Geometry check sheet. Reference: the model listing, model coordinates, mm. Face numbers are marked on the shaded views. A direction names the side the tool comes from. Give positions to 0.01 mm unless a question says otherwise; leave off trailing zeros. Order: outer loops, then holes, each group sorted by start corner. A loop starts at its lowest first (then second) coordinate and runs counter-clockwise, first axis right, second up. Notation, with made-up numbers: M 64,-0.5 L 114,-0.5 A10 cw 114,17.5 Z; hole C 80,78.5 d8. An arc over 180 degrees is marked long. Put each result on its own line as item: value. Start each with the question number.
Q1. Material ranges on L1, parallel to X at y = 10.75, z = 9.5; L2, parallel to Z at x = -13, y = 10; L3, parallel to X at y = 8.25, z = 7.75, recorded low to high.
Q2. Mould release check, pull along X, two halves, no side actions. Record for the marked faces 1, 2 and 3: +X half, -X half, draft (parallel to the pull), parting line (faces both ways), or undercut.
Q3. Go/stop test with flat-tipped pins: pin 1 (5.5 mm diameter, centred on x = 12, y = 5, fed in from +Z); pin 2 (2 mm diameter, centred on y = 8, z = 7, fed in from +X); pin 3 (4 mm diameter, centred on y = 4, z = 8, fed in from -X). Record where each tip stops, or that it passes through.
Q4. Section check A-A on z = 10.5. Record the cut outline in (x, y).
Q5. Section check D-D on y = 5. Record the cut outline in (x, z), then the cut area to 4 significant figures.
Q6. Section check B-B on x = -14. Record the cut outline in (y, z), then the cut area to 3 significant figures.
Q7. Section check C-C on y = 9.75. Record the cut outline in (x, z).
Q8. Access from +Z, -Z, +X, -X, +Y, -Y to the whole of each face (thin tool, end or side, straight path). Record for the marked faces 4, 5 and 6.
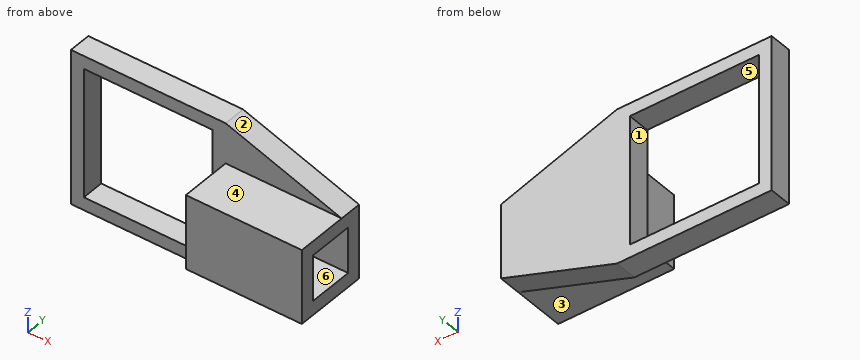
Autodesk Fusion 360 part; units mm, degrees
sketch "Sketch1" plane through (0, 0, 0) normal (0, 1, 0) x (1, 0, 0)
  line L0 (0, 0) -> (0, -11.5)
  line L1 (0, -11.5) -> (18, -11.5)
  line L2 (0, 0) -> (18, 0)
  line L3 (18, -11.5) -> (18, 0)
  dimension "d1" = 11.5
  dimension "d2" = 18
  dimension "d3" = 18
extrude "Extrude1" add sketch "Sketch1" along normal blind 11.5
sketch "Sketch2" plane through (18, 0, 0) normal (1, 0, 0) x (0, 1, 0)
  line L0 (0, 11.5) -> (0, 0)
  line L1 (0, 0) -> (11.5, 0)
  line L2 (11.5, 0) -> (11.5, 11.5)
  line L3 (11.5, 11.5) -> (0, 11.5)
  line L4 (0, 11.5) -> (0, 9.3)
  line L5 (0, 9.3) -> (2.2, 9.3)
  line L6 (2.2, 9.3) -> (9.3, 9.3)
  line L7 (9.3, 9.3) -> (9.3, 2.2)
  line L8 (9.3, 2.2) -> (2.2, 2.2)
  line L9 (2.2, 2.2) -> (2.2, 9.3)
  dimension "d9" = 2.2
  dimension "d10" = 2.2
  dimension "d11" = 7.1
  dimension "d12" = 7.1
extrude "Extrude2" cut sketch "Sketch2" against normal blind 15 contours L6 L7 L8 L9
sketch "Sketch3" plane through (0, 0, 0) normal (-1, 0, 0) x (0, -1, 0)
  line L0 (0, 0) -> (0, 11.5)
  line L1 (0, 11.5) -> (-11.5, 11.5)
  line L2 (-11.5, 11.5) -> (-11.5, 0)
  line L3 (-11.5, 0) -> (0, 0)
  line L4 (-11.5, 11.5) -> (-7.25, 11.5)
  line L5 (-7.25, 11.5) -> (-7.25, 7.25)
  line L6 (-7.25, 7.25) -> (-4.25, 7.25)
  line L7 (-4.25, 7.25) -> (-4.25, 4.25)
  line L8 (-4.25, 4.25) -> (-7.25, 4.25)
  line L9 (-7.25, 4.25) -> (-7.25, 7.25)
  dimension "d15" = 4.25
  dimension "d16" = 4.25
  dimension "d17" = 3
  dimension "d18" = 3
sketch "Sketch4" plane through (0, 0, 0) normal (-1, 0, 0) x (0, -1, 0)
  line L0 (0, 0) -> (0, 11.5)
  line L1 (0, 11.5) -> (-11.5, 11.5)
  line L2 (-11.5, 11.5) -> (-11.5, 0)
  line L3 (-11.5, 0) -> (0, 0)
  line L4 (-11.5, 11.5) -> (-11.5, 7.5)
  line L5 (-11.5, 7.5) -> (0, 7.5)
  line L6 (0, 7.5) -> (0, 4)
  line L7 (0, 4) -> (-11.5, 4)
  line L8 (-11.5, 4) -> (-11.5, 7.5)
  dimension "d21" = 4
  dimension "d22" = 3.5
sketch "Sketch5" plane through (0, 0, 0) normal (0, -1, 0) x (1, 0, 0)
  line L0 (0, 11.5) -> (0, 0)
  line L1 (0, 0) -> (18, 0)
  line L2 (18, 0) -> (18, 11.5)
  line L3 (18, 11.5) -> (0, 11.5)
  line L4 (0, 11.5) -> (0, 0)
sketch "Sketch6" plane through (0, 11.5, 0) normal (0, 1, 0) x (-1, 0, 0)
  line L0 (0, 0) -> (0, 11.5)
  line L1 (0, 11.5) -> (-18, 11.5)
  line L2 (-18, 11.5) -> (-18, 0)
  line L3 (-18, 0) -> (0, 0)
  line L4 (0, 5.75) -> (24, 5.75)
  line L5 (24, 5.75) -> (24, 17.75)
  line L6 (24, 17.75) -> (0, 17.75)
  line L7 (0, 17.75) -> (0, 5.75)
  line L8 (0, 5.75) -> (-18, 5.75) construction
  line L9 (24, 5.75) -> (24, -6.25)
  line L10 (24, -6.25) -> (0, -6.25)
  line L11 (0, 5.75) -> (24, 5.75)
  line L12 (0, -6.25) -> (0, 0)
  dimension "d26" = 24
  dimension "d27" = 12
extrude "Extrude5" add sketch "Sketch6" against normal blind 3.5 contours L0 L4 L9 L10 L11 L12 | L0 L4 L5 L6 L7 L11
sketch "Sketch7" plane through (0, 11.5, 0) normal (0, 1, 0) x (-1, 0, 0)
  line L0 (0, 11.5) -> (-18, 11.5)
  line L1 (-18, 11.5) -> (-18, 0)
  line L2 (-18, 0) -> (0, 0)
  line L3 (0, 0) -> (0, -6.25)
  line L4 (0, -6.25) -> (24, -6.25)
  line L5 (24, -6.25) -> (24, 17.75)
  line L6 (24, 17.75) -> (0, 17.75)
  line L7 (0, 17.75) -> (0, 11.5)
  line L8 (24, -6.25) -> (24, -4.25)
  line L9 (24, -4.25) -> (22, -4.25)
  line L10 (22, -4.25) -> (2, -4.25)
  line L11 (2, -4.25) -> (2, 15.75)
  line L12 (2, 15.75) -> (22, 15.75)
  line L13 (22, 15.75) -> (22, -4.25)
  dimension "d30" = 2
  dimension "d31" = 2
  dimension "d32" = 20
  dimension "d33" = 20
extrude "Extrude6" cut sketch "Sketch7" against normal blind 5 contours L10 L11 L12 L13
sketch "Sketch8" plane through (0, 0, 0) normal (1, 0, 0) x (0, 1, 0)
sketch "Sketch9" plane through (0, 11.5, 0) normal (0, 1, 0) x (-1, 0, 0)
  line L0 (2, -4.25) -> (2, 15.75)
  line L1 (2, 15.75) -> (22, 15.75)
  line L2 (22, 15.75) -> (22, -4.25)
  line L3 (22, -4.25) -> (2, -4.25)
  line L4 (0, 11.5) -> (-18, 11.5)
  line L5 (-18, 11.5) -> (-18, 0)
  line L6 (-18, 0) -> (0, 0)
  line L7 (0, 0) -> (0, -6.25)
  line L8 (0, -6.25) -> (24, -6.25)
  line L9 (24, -6.25) -> (24, 17.75)
  line L10 (24, 17.75) -> (0, 17.75)
  line L11 (0, 17.75) -> (0, 11.5)
  line L12 (0, -6.25) -> (-18, 0)
  line L13 (0, 17.75) -> (-18, 11.5)
extrude "Extrude7" add sketch "Sketch9" against normal blind 3.5 contours L4 L11 L13 | L6 L7 L12
Results found:
1. L1: x = -24 to -22, -2 to 18
1. L2: z = -6.25 to -4.25, 15.75 to 17.75
1. L3: x = -24 to -22, -2 to 3
2. face 1: undercut
2. face 2: +X half
2. face 3: draft
3. pin 1: stops at z = 11.5
3. pin 2: stops at x = 3
3. pin 3: stops at x = 0
4. outline: M -24,8 L -22,8 L -22,11.5 L -24,11.5 Z; M -2,8 L 0,8 L 0,0 L 18,0 L 18,11.5 L -2,11.5 Z
5. outline: M 0,0 L 18,0 L 18,2.2 L 3,2.2 L 3,9.3 L 18,9.3 L 18,11.5 L 0,11.5 Z
5. area: 100.5 mm^2
6. outline: M 8,-6.25 L 11.5,-6.25 L 11.5,-4.25 L 8,-4.25 Z; M 8,15.75 L 11.5,15.75 L 11.5,17.75 L 8,17.75 Z
6. area: 14.0 mm^2
7. outline: M -24,-6.25 L 0,-6.25 L 18,0 L 18,11.5 L 0,17.75 L -24,17.75 Z; hole M -22,-4.25 L -2,-4.25 L -2,15.75 L -22,15.75 Z
8. face 4: +Z, +X, -X, -Y
8. face 5: +Y, -Y
8. face 6: +X
